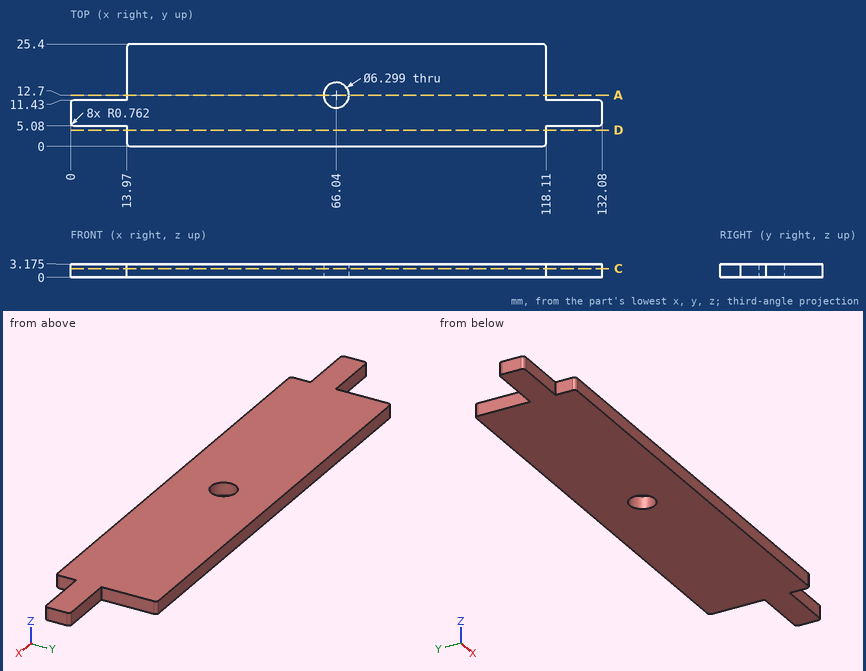
Source: three-view drawing plus pictorial views. Frame: mm from the lowest corner of the part. Round coordinates to 2 decimals unless told otherwise and drop trailing zeros. Order: outer loops, then holes, each group sorted by start corner. A loop starts at its lowest first (then second) coordinate and runs counter-clockwise, first axis right, second up. Notation, with made-up numbers: (-14, 44) -> (26, 44) arc R18 cw to (26, 59) -> close; hole circle Ø10 at (36, -3). An arc over 180 degrees is marked (long way). Use one line per item in the form item = value. Start each with the question number.
1. Pin query (flat end, axial travel): pin 1 Ø1.6 at (y, z) = (18, 2) entering from +X; pin 2 Ø1.6 at (x, z) = (9, 1) entering from -Y; pin 3 Ø8 at (x, y) = (66.04, 12.7) entering from -Z; pin 4 Ø1.6 at (y, z) = (15.5, 2) entering from -X. Return the tip coordinate at first contact, or that it passes through.
2. Cut plane C-C (z = 2.1). Return the cut outline in (x, y), then the cut area to 3 significant figures.
3. Cut plane A-A (y = 12.7). Return the cut outline in (x, z) (1 decimal).
4. Line query: probe 1 along Y at (x, z) = (66.04, 0.9); probe 2 along X at (y, z) = (12.5, 1.5); probe 3 along X at (y, z) = (17.25, 0.9). Output: solid intervals per line, ascending.
5. Cut plane D-D (y = 4). Return the cut outline in (x, z) (3 decimals), then the cut area to 3 significant figures.
Solution:
q1.pin_1 = 118.11
q1.pin_2 = 5.08
q1.pin_3 = 0
q1.pin_4 = 13.97
q2.outline = (0, 5.84) arc R0.76 ccw to (0.76, 5.08) -> (13.97, 5.08) -> (13.97, 0.76) arc R0.76 ccw to (14.73, 0) -> (117.35, 0) arc R0.76 ccw to (118.11, 0.76) -> (118.11, 5.08) -> (131.32, 5.08) arc R0.76 ccw to (132.08, 5.84) -> (132.08, 10.67) arc R0.76 ccw to (131.32, 11.43) -> (118.11, 11.43) -> (118.11, 24.64) arc R0.76 ccw to (117.35, 25.4) -> (14.73, 25.4) arc R0.76 ccw to (13.97, 24.64) -> (13.97, 11.43) -> (0.76, 11.43) arc R0.76 ccw to (0, 10.67) -> close; hole circle Ø6.3 at (66.04, 12.7)
q2.area = 2,790 mm^2
q3.outline = (14, 0) -> (62.9, 0) -> (62.9, 3.2) -> (14, 3.2) -> close; (69.2, 0) -> (118.1, 0) -> (118.1, 3.2) -> (69.2, 3.2) -> close
q4.probe_1 = 0 to 9.55, 15.85 to 25.4
q4.probe_2 = 13.97 to 62.9, 69.18 to 118.11
q4.probe_3 = 13.97 to 118.11
q5.outline = (13.97, 0) -> (118.11, 0) -> (118.11, 3.175) -> (13.97, 3.175) -> close
q5.area = 331 mm^2
